Autodesk Inventor part; units mm, degrees
ref_plane "YZ Plane" through (0, 0, 0) normal (1, 0, 0) x (0, 1, 0)
ref_plane "XZ Plane" through (0, 0, 0) normal (0, 1, 0) x (-1, 0, 0)
ref_plane "XY Plane" through (0, 0, 0) normal (0, 0, 1) x (1, 0, 0)
sketch "Sketch2" plane through (0, 0, 0) normal (1, 0, 0) x (0, 0, -1)
  circle A0 centre (0, 0) radius 14.2875
  arc A1 (25.4, 0) -> (-25.4, 0) centre (0, 0) ccw
  line L0 (-25.4, 0) -> (-25.4, -25.4)
  line L1 (25.4, 0) -> (25.4, -25.4)
  arc A2 (-71.9234, -86.0305) -> (-25.4, -25.4) centre (-88.1693, -25.4) ccw
  arc A3 (-58.7754, -135.0995) -> (25.4, -25.4) centre (-88.1693, -25.4) ccw
  line L2 (-88.1693, -25.4) -> (-58.7754, -135.0995) construction
  line L3 (-71.9234, -86.0305) -> (-133.2597, -102.4655)
  line L4 (-58.7754, -135.0995) -> (-120.1117, -151.5345)
  arc A4 (-133.2597, -102.4655) -> (-120.1117, -151.5345) centre (-126.6857, -127) ccw
  circle A5 centre (-126.6857, -127) radius 14.2875
  line L5 (-88.1693, -25.4) -> (25.4, -25.4) construction
  dimension "d0" = 28.575
  dimension "d1" = 25.4
  dimension "d2" = 28.575
  dimension "d3" = 25.4
  dimension "d4" = 63.5
  dimension "d5" = 127
  dimension "d6" = 75
extrude "Extrusion1" add sketch "Sketch2" along normal blind 6.35
properties part number "Claw"
Geometry: final body of the model. Coordinates: model frame, mm. Coordinates: 2 decimals unless noted, no trailing zeros. Order: outer loops, then holes, each group sorted by start corner. A loop starts at its lowest first (then second) coordinate and runs counter-clockwise, first axis right, second up.
(1) Section query D-D (y = -47.5). Return the cut outline in (x, z), plus the area to 3 significant figures.
(2) Draft query along Z for faces 1 (the face through (3.1, -121.5, 113.5)), 2 (the face through (3, -13, -25.4)), 3 (the face through (3, -13, 25.4)). Return one class per face: pulls with the +Z half, pulls with the -Z half, needs draft (parallel to the pull), parting line crosses it, or undercut.
(3) Section query C-C (z = 0). Return the cut outline in (x, y).
(4) Section query A-A (x = 5). Return the cut outline in (y, z) (1 decimal), plus the area to 3 significant figures.
(5) Section query B-B (y = 3.5). Return the cut outline in (x, z).
(6) Material intervals for probe 1 along Z at (x, y) = (5.5, -122.5); probe 2 along Y at (x, z) = (3.5, -0.5); probe 3 along Y at (x, z) = (4.75, -3.5), sorted ascending.
(7) First-contact query: pin 1 (1.9 mm diameter, centred on x = 3, y = -17, fed in from +Z); pin 2 (3 mm diameter, centred on x = 2, y = -88.5, fed in from -Z); pin 3 (2 mm diameter, centred on x = 3, z = 74.5, fed in from +Y). Flat tips, straight axial feed; report the tip coordinate or a pass-through.
Solution:
1. outline: (0, -23.23) - (6.35, -23.23) - (6.35, 29.42) - (0, 29.42) - close
1. area: 334 mm2
2. face 1: undercut
2. face 2: pulls with the -Z half
2. face 3: pulls with the +Z half
3. outline: (0, -96.98) - (6.35, -96.98) - (6.35, -14.29) - (0, -14.29) - close; (0, 14.29) - (6.35, 14.29) - (6.35, 25.4) - (0, 25.4) - close
4. outline: (-151.5, 120.1) - (-135.1, 58.8) arc R113.6 ccw to (-25.4, -25.4) - (0, -25.4) arc R25.4 ccw to (0, 25.4) - (-25.4, 25.4) arc R62.8 cw to (-86, 71.9) - (-102.5, 133.3) arc R25.4 ccw to start; hole circle Ø28.6 at (-127, 126.7); hole circle Ø28.6 at (0, 0)
4. area: 11,100 mm2
5. outline: (0, -25.16) - (6.35, -25.16) - (6.35, -13.85) - (0, -13.85) - close; (0, 13.85) - (6.35, 13.85) - (6.35, 25.16) - (0, 25.16) - close
6. probe 1: z = 29.27 to 113.13, 140.25 to 151.68
6. probe 2: y = -96.36 to -14.28, 14.28 to 25.4
6. probe 3: y = -92.44 to -13.85, 13.85 to 25.16
7. pin 1: stops at z = 25.4
7. pin 2: stops at z = -7.24
7. pin 3: stops at y = -86.45
